Part model, mm, in its own coordinate system. A direction names the side the tool comes from. Coordinates: 2 decimals unless noted, no trailing zeros. Loops run counter-clockwise (first coordinate to the right, second up) from the corner with the lowest first, then second, coordinate; pieces in that order, holes last. Notation, with made-up numbers: M 45,7.25 L 50,7.25 A24 ccw 50,25.25 Z; hole C 56,44.25 d10. An arc over 180 degrees is marked long. Answer as CSV lines item,"result". Start each with the question number.
from build123d import *

# Parameters (mm, degrees)
BOSS_EXTRUDE1_DEPTH = 4
FILLET1_R           = 0.4
FILLET2_R           = 0.6


with BuildPart() as part:
    # Sketch1 → Boss-Extrude1 (new body)
    with BuildSketch(Plane.XY):
        with BuildLine():
            Line((-14.499129977, -6.867012113), (14.367174161, -16))
            Line((14.367174161, -16), (18.15387109, -16))
            ThreePointArc((18.15387109, -16), (25.872793622, -19.642466284), (27.968533139, -27.91635301))
            Line((27.968533139, -27.91635301), (27.439499229, -30.625816775))
            ThreePointArc((27.439499229, -30.625816775), (26.748073563, -31.786330679), (25.476566819, -32.242546173))
            Line((25.476566819, -32.242546173), (18, -32.242546173))
            Line((18, -32.242546173), (18, -36.892546173))
            Line((18, -36.892546173), (23.78761885, -36.892546173))
            ThreePointArc((23.78761885, -36.892546173), (25.331403357, -37.62103943), (25.75055126, -39.275816775))
            Line((25.75055126, -39.275816775), (19.168328866, -72.986875227))
            ThreePointArc((19.168328866, -72.986875227), (18.903762814, -78.877039551), (20.368176295, -84.588390014))
            Line((20.368176295, -84.588390014), (30.173934909, -107.85))
            Line((30.173934909, -107.85), (24.678215229, -107.85))
            Line((24.678215229, -107.85), (24.678215229, -111.75))
            Line((24.678215229, -111.75), (31.817950891, -111.75))
            Line((31.817950891, -111.75), (49.494630027, -153.683320214))
            Line((49.494630027, -153.683320214), (39.586931175, -157.859836948))
            Line((39.586931175, -157.859836948), (41.101848885, -161.453584898))
            Line((41.101848885, -161.453584898), (51.009547737, -157.277068164))
            Line((51.009547737, -157.277068164), (59.688079015, -177.864624701))
            ThreePointArc((59.688079015, -177.864624701), (62.10799078, -184.18292059), (64.103704557, -190.647745599))
            Line((64.103704557, -190.647745599), (52.448848585, -197.218781175))
            Line((52.448848585, -197.218781175), (65.808694789, -197.945888914))
            Line((65.808694789, -197.945888914), (53.567462973, -203.346483316))
            Line((53.567462973, -203.346483316), (66.884945667, -204.634439433))
            Line((66.884945667, -204.634439433), (54.312217418, -209.210538279))
            Line((54.312217418, -209.210538279), (67.514830834, -211.379679878))
            Line((67.514830834, -211.379679878), (54.666068058, -215.111096686))
            Line((54.666068058, -215.111096686), (67.695571684, -218.151855063))
            Line((67.695571684, -218.151855063), (54.627453954, -221.022129484))
            Line((54.627453954, -221.022129484), (67.42637092, -224.921090983))
            Line((67.42637092, -224.921090983), (54.196545445, -226.917561415))
            Line((54.196545445, -226.917561415), (66.708416062, -231.657526599))
            Line((66.708416062, -231.657526599), (53.375243393, -232.771386039))
            Line((53.375243393, -232.771386039), (65.544874215, -238.331445565))
            Line((65.544874215, -238.331445565), (52.167170795, -238.557780459))
            Line((52.167170795, -238.557780459), (63.940878095, -244.913407312))
            Line((63.940878095, -244.913407312), (50.577656806, -244.251219233))
            Line((50.577656806, -244.251219233), (61.903503389, -251.374376921))
            Line((61.903503389, -251.374376921), (48.613713227, -249.826586971))
            Line((48.613713227, -249.826586971), (59.44173754, -257.685853206))
            Line((59.44173754, -257.685853206), (46.284003576, -255.259289128))
            Line((46.284003576, -255.259289128), (56.566440102, -263.819994437))
            Line((56.566440102, -263.819994437), (43.59880487, -260.525360501))
            Line((43.59880487, -260.525360501), (53.290294836, -269.749741158))
            Line((53.290294836, -269.749741158), (40.569962289, -265.601570939))
            Line((40.569962289, -265.601570939), (49.627753757, -275.448935561))
            ThreePointArc((49.627753757, -275.448935561), (28.558785484, -297.812941794), (1.785859605, -312.888108085))
            Line((1.785859605, -312.888108085), (-3.79713943, -315))
            ThreePointArc((-3.79713943, -315), (-33.79713943, -294.273546964), (-25.025440375, -258.880847842))
            Line((-25.025440375, -258.880847842), (-19.44244134, -256.768955927))
            ThreePointArc((-19.44244134, -256.768955927), (4.29821428, -234.038615683), (4.399649005, -201.171051004))
            Line((4.399649005, -201.171051004), (-16.026093015, -152.716294646))
            ThreePointArc((-16.026093015, -152.716294646), (-22.647715731, -129.865425568), (-23.795753165, -106.102216294))
            Line((-23.795753165, -106.102216294), (-19.167544676, -38.755425513))
            ThreePointArc((-19.167544676, -38.755425513), (-18.537124111, -37.430656759), (-17.172250732, -36.892546173))
            Line((-17.172250732, -36.892546173), (-5.905128728, -36.892546173))
            Line((-5.905128728, -36.892546173), (-7.597590317, -32.242546173))
            Line((-7.597590317, -32.242546173), (-16.577805132, -32.242546173))
            ThreePointArc((-16.577805132, -32.242546173), (-18.039694546, -31.607419552), (-18.573099077, -30.105425513))
            Line((-18.573099077, -30.105425513), (-17.975910939, -21.415517819))
            Line((-17.975910939, -21.415517819), (-11.538306364, -21.415517819))
            Line((-11.538306364, -21.415517819), (-13.230767953, -16.765517819))
            Line((-13.230767953, -16.765517819), (-17.656353478, -16.765517819))
            Line((-17.656353478, -16.765517819), (-17.097726509, -8.636728098))
            ThreePointArc((-17.097726509, -8.636728098), (-16.228213916, -7.12078604), (-14.499129977, -6.867012113))
        make_face()
        with BuildLine():
            Line((-8.039189398, -14.802148248), (-6.329088682, -19.500611352))
            ThreePointArc((-6.329088682, -19.500611352), (-5.759253375, -20.395073615), (-4.864791112, -20.964908922))
            Line((-4.864791112, -20.964908922), (9.662050649, -26.252246921))
            ThreePointArc((9.662050649, -26.252246921), (11.905262269, -25.956922509), (12.95, -23.95))
            Line((12.95, -23.95), (12.95, -19.101392708))
            ThreePointArc((12.95, -19.101392708), (12.476507259, -17.653663778), (11.23904567, -16.765517819))
            Line((11.23904567, -16.765517819), (-4.997896808, -11.628324008))
            ThreePointArc((-4.997896808, -11.628324008), (-7.505894036, -12.269114715), (-8.039189398, -14.802148248))
        make_face(mode=Mode.SUBTRACT)
        with BuildLine():
            Line((-1.8643328, -31.767427321), (3.165925841, -45.587949351))
            ThreePointArc((3.165925841, -45.587949351), (4.062910493, -46.756922509), (5.468172762, -47.2))
            Line((5.468172762, -47.2), (10.5, -47.2))
            ThreePointArc((10.5, -47.2), (12.232411614, -46.482411614), (12.95, -44.75))
            Line((12.95, -44.75), (12.95, -34.591777725))
            ThreePointArc((12.95, -34.591777725), (12.506922509, -33.186515456), (11.337949351, -32.289530804))
            Line((11.337949351, -32.289530804), (1.275863472, -28.627231049))
            ThreePointArc((1.275863472, -28.627231049), (-1.294497493, -29.197066356), (-1.8643328, -31.767427321))
        make_face(mode=Mode.SUBTRACT)
        with BuildLine():
            Line((1.657284816, -78.8176291), (10.596301358, -100.023119123))
            ThreePointArc((10.596301358, -100.023119123), (10.419751266, -101.905947161), (8.753353691, -102.8))
            Line((8.753353691, -102.8), (-6.141789596, -102.8))
            ThreePointArc((-6.141789596, -102.8), (-7.654833819, -102.107936229), (-8.120754951, -100.510697178))
            ThreePointArc((-8.120754951, -100.510697178), (-8.05444857, -100.065191098), (-7.985836627, -99.620034266))
            ThreePointArc((-7.985836627, -99.620034266), (-7.962968981, -99.498759801), (-7.932665095, -99.379126613))
            Line((-7.932665095, -99.379126613), (-2.108355103, -79.043824493))
            ThreePointArc((-2.108355103, -79.043824493), (-0.305583194, -77.598108436), (1.657284816, -78.8176291))
        make_face(mode=Mode.SUBTRACT)
        with BuildLine():
            Line((-3.521215631, -298.858320046), (-6.119790114, -299.841287875))
            ThreePointArc((-6.119790114, -299.841287875), (-19.76735139, -288.966471728), (-16.733940587, -271.781711796))
            Line((-16.733940587, -271.781711796), (-14.135366104, -270.798743967))
            ThreePointArc((-14.135366104, -270.798743967), (18.084095095, -239.950425064), (18.221756508, -195.344444428))
            Line((18.221756508, -195.344444428), (-14.560581286, -117.576880877))
            ThreePointArc((-14.560581286, -117.576880877), (-13.741730826, -115.082087048), (-11.157717662, -115.548336225))
            Line((-11.157717662, -115.548336225), (47.774811887, -188.994412647))
            ThreePointArc((47.774811887, -188.994412647), (47.968900833, -189.285104624), (48.109417057, -189.605147645))
            ThreePointArc((48.109417057, -189.605147645), (44.356574969, -254.657971176), (-3.521215631, -298.858320046))
        make_face(mode=Mode.SUBTRACT)
    extrude(amount=BOSS_EXTRUDE1_DEPTH)

    # Fillet1
    fillet1_edges = [part.edges().sort_by_distance(p)[0] for p in [
        (64.103704557, -190.647745599, 2),
        (49.627753757, -275.448935561, 2),
        (40.569962289, -265.601570939, 2),
        (43.59880487, -260.525360501, 2),
        (46.284003576, -255.259289128, 2),
        (48.613713227, -249.826586971, 2),
        (50.577656806, -244.251219233, 2),
        (52.167170795, -238.557780459, 2),
        (53.375243393, -232.771386039, 2),
        (54.196545445, -226.917561415, 2),
        (54.627453954, -221.022129484, 2),
        (54.666068058, -215.111096686, 2),
        (54.312217418, -209.210538279, 2),
        (53.567462973, -203.346483316, 2),
        (52.448848585, -197.218781175, 2),
    ]]
    fillet(fillet1_edges, radius=FILLET1_R)

    # Fillet2
    fillet2_edges = [part.edges().sort_by_distance(p)[0] for p in [
        (53.290294836, -269.749741158, 2),
        (56.566440102, -263.819994437, 2),
        (59.44173754, -257.685853206, 2),
        (61.903503389, -251.374376921, 2),
        (63.940878095, -244.913407312, 2),
        (65.544874215, -238.331445565, 2),
        (66.708416062, -231.657526599, 2),
        (67.42637092, -224.921090983, 2),
        (67.695571684, -218.151855063, 2),
        (67.514830834, -211.379679878, 2),
        (66.884945667, -204.634439433, 2),
        (65.808694789, -197.945888914, 2),
    ]]
    fillet(fillet2_edges, radius=FILLET2_R)


solid = part.part
Q1. Tool access for faces 4 (the face through (58.809, -193.633, 1.972)), 5 (the face through (2.297, -23.572, 1.972)), 6 (the face through (-7, -159, 0)), 7 (the face through (-5.67, -177.28, 1.97)): list every direction of +Z, -Z, +X, -X, +Y, -Y with a clear straight run to the whole face (end or side of a thin tool).
Q2. Flat gauge pins, fed straight in: P1, Ø1, axis at x = 15, z = 3.5, coming from the +Y side; P2, Ø2, axis at y = -103.5, z = 1, coming from the -X side; P3, Ø1.2, axis at y = -40, z = 1, coming from the -X side. Where does each tip first touch, or does it go through?
Q3. Two-plate mould, pull along Y, no slides. Class faces 1 (the face through (17.9, -151.76, 1.97)), 2 (the face through (-7, -159, 4)), 3 (the face through (-33.6, -294.78, 1.97)): +Y half, -Y half, draft (parallel to the pull), parting line (faces both ways), or undercut.
Q4. Slice it at A-A, the plane y = -88.5. Write the cut outline in (x, z), and give its area (3 significant figures).
Q5. Slice it at C-C, the plane y = -132.5. Write the cut outline in (x, z), and give its area (3 significant figures).
Q6. Slice it at B-B, the plane z = 1.05. State how many separate pieces and enclosed holes the cut face has, and give its area (3 significant figures).
Q7. Wall check: L1, parallel to Y at x = -9, z = 2.45; L2, parallel to Y at x = 16, z = 2.85; L3, parallel to X at y = -296, z = 2.4. Give the ranges that are in metal, low to high.
Solved:
1,face 4,"+Z, -Z, +X"
1,face 5,"+Z, -Z"
1,face 6,"-Z, +X, -X, +Y, -Y"
1,face 7,"+Z, -Z, -X"
2,P1,"stops at y = -16"
2,P2,"stops at x = -23.69"
2,P3,"stops at x = -19.29"
3,face 1,"undercut"
3,face 2,"draft"
3,face 3,"parting line"
4,outline,"M -22.59,0 L -4.82,0 L -4.82,4 L -22.59,4 Z; M 5.74,0 L 22.02,0 L 22.02,4 L 5.74,4 Z"
4,area,"136 mm2"
5,outline,"M -22.17,0 L -8.27,0 L -8.27,4 L -22.17,4 Z; M 2.44,0 L 40.56,0 L 40.56,4 L 2.44,4 Z"
5,area,"208 mm2"
6,separate pieces,"1"
6,enclosed holes,"4"
6,area,"11,000 mm2"
7,L1,"y = -314.58 to -299.19, -268.56 to -251.01, -169.38 to -130.77, -118.24 to -36.89, -32.24 to -8.61"
7,L2,"y = -306.22 to -288.47, -244.29 to -190.07, -149.39 to -16"
7,L3,"x = -33.09 to -14.78, 3.17 to 30.81"
